Read the model definition and answer for the solid it produces. Units are mm, in the model's axes. A direction names the side the tool comes from. Coordinates: 2 decimals unless noted, no trailing zeros. Loops run counter-clockwise (first coordinate to the right, second up) from the corner with the lowest first, then second, coordinate; pieces in that order, holes last.
from build123d import *

# Parameters (mm, degrees)
F0_W      = 26
F0_H      = 26
F0_W_2    = 22
F0_H_2    = 22
F1_DEPTH  = 75
F5_DEPTH  = 26.001
F9_DEPTH  = 44.548727
F11_DEPTH = 26.001


with BuildPart() as f1:
    # F0 (on Top) → F1 (new body)
    with BuildSketch(Plane.XY):
        Rectangle(F0_W, F0_H)
        Rectangle(F0_W_2, F0_H_2, mode=Mode.SUBTRACT)
    extrude(amount=F1_DEPTH)

    # F2 (on face) → F5 (cut, through all)
    with BuildSketch(Plane.XZ.offset(13)):
        Polygon((13, 26), (-13, 0), (13, 0), align=None)
    extrude(amount=-F5_DEPTH, mode=Mode.SUBTRACT)

    # F8 (on face) → F9 (cut, through all)
    with BuildSketch(Plane(origin=(-12.5, 0, 12.5), x_dir=(0, 1, 0), z_dir=(0.707107, 0, -0.707107))):
        Polygon((-13, 47.179355), (-6.58165, 36.062446), (13, 47.367917), (13, 69.708109), (-13, 69.708109), align=None)
    extrude(amount=-F9_DEPTH, mode=Mode.SUBTRACT)

    # F10 (on face) → F11 (cut, through all)
    with BuildSketch(Plane.XZ.offset(13)):
        Polygon((-13, 87.199546), (-13, 50), (20.817262, 83.817262), (20.817262, 87.199546), align=None)
    extrude(amount=-F11_DEPTH, mode=Mode.SUBTRACT)


solid = f1.part
Item 1: A cutting plane is placed at C-C on y = 9.5. Determine the outline of the cut face in (x, z), then the cut area to 3 significant figures.
Numbers:
outline: (-13, 0) - (-11, 2) - (-11, 52) - (-13, 50) - close; (11, 24) - (13, 26) - (13, 51.13) - (11, 53.13) - close
area: 154 mm2
Item 2: Find the intervals of material crossed by line 1 along X through (y, z) = (-3.5, 32.5); line 2 along X through (y, z) = (-6.25, 47.5), in increasing order.
Numbers:
line 1: x = -13 to -11, 11 to 13
line 2: x = -13 to -11
Item 3: A cutting plane is placed at A-A on z = 29.5. Determine the outline of the cut face in (x, y).
Numbers:
outline: (-13, -13) - (13, -13) - (13, 13) - (-13, 13) - close; hole (-11, -11) - (11, -11) - (11, 11) - (-11, 11) - close
Item 4: Determine the mould class of faces 1 (the face through (0, -13, 32)), 2 (the face through (-11, 0, 27)), 3 (the face through (-12, 0, 51)) for opening direction Y: released by +Y, released by -Y, zero draft, split by the parting line, or undercut.
Numbers:
face 1: released by -Y
face 2: undercut
face 3: zero draft
Item 5: A cutting plane is placed at B-B on x = -3.25. Determine the outline of the cut face in (y, z), then the cut area to 3 significant figures.
Numbers:
outline: (-13, 9.75) - (-11, 9.75) - (-11, 59.75) - (-13, 59.75) - close; (11, 9.75) - (13, 9.75) - (13, 59.75) - (11, 59.75) - close
area: 200 mm2
Item 6: A cutting plane is placed at D-D on z = 14. Determine the outline of the cut face in (x, y), then the cut area to 3 significant figures.
Numbers:
outline: (-13, -13) - (1, -13) - (1, -11) - (-11, -11) - (-11, 11) - (1, 11) - (1, 13) - (-13, 13) - close
area: 100 mm2
Item 7: Given pin 1 (10 mm diameter, centred on x = -1.5, y = 8, fed in from -Z); pin 2 (12 mm diameter, centred on x = 5, y = 6.5, fed in from +Z), each flat-ended and moving along its own axis, determine where each tip first touches the part or whether it passes through.
Numbers:
pin 1: stops at z = 7.5
pin 2: stops at z = 64.25
Item 8: Which of the six approach directions +Z, -Z, +X, -X, +Y, -Y give full straight-line access (tool end or side, diameter ignored) to faces 4 (the face through (0, -11, 32)), 5 (the face through (11.4, 7.5, 51.1)), 6 (the face through (13, 0, 37))?
Numbers:
face 4: +Z, -Z
face 5: +Z, +X
face 6: +Z, -Z, +X, +Y, -Y
